Verification items for this drawing (mm, ordinates from the low corner). Coordinates: 2 decimals unless noted, no trailing zeros. Write each loop counter-clockwise with the first axis right and the second up, starting at its lowest first coordinate (ties: lowest second). Pieces come first, ordered by that corner, then holes. Notation, with made-up numbers: (58.5, -21) -> (89.5, -21) arc R26 ccw to (89.5, 7) -> close; hole circle Ø6 at (-15.5, 39). An arc over 180 degrees is marked (long way). Put each result on its own line as item: value. Start each with the question number.
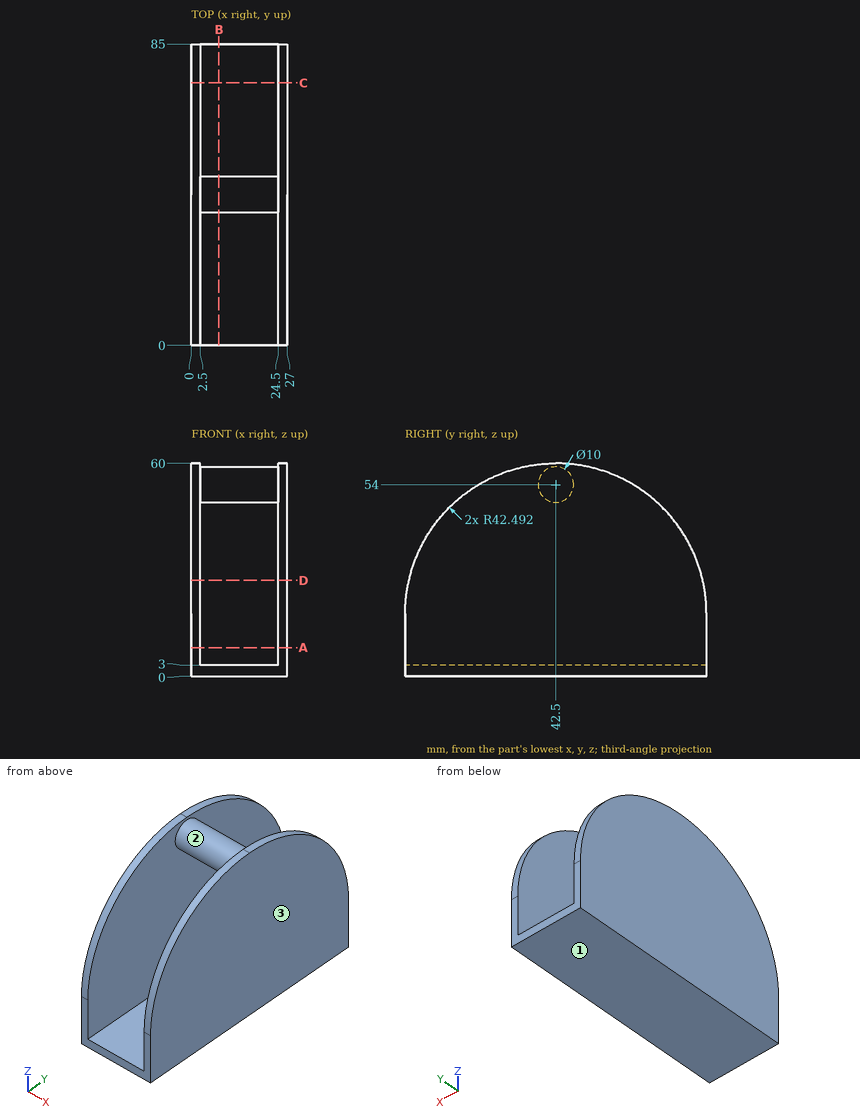
Item 1: Mould release check, pull along Z, two halves, no side actions. Record for the marked faces 1, 2 and 3: released by +Z, released by -Z, zero draft, split by the parting line, or undercut.
Item 2: Scan lines: line 1 along X through (y, z) = (31.5, 54.5); line 2 along Z through (x, y) = (19, 14.5); line 3 along Z through (x, y) = (6.75, 44). Record each from-to range of solid material in increasing order. Write a range as [from, to].
Item 3: Section check D-D, the plane z = 27. Enter the section's corners in (x, y).
Item 4: Section check A-A, the plane z = 8. Enter the section's corners in (x, y), and give its area (3 significant figures).
Item 5: Section check C-C, the plane y = 74. Enter the section's corners in (x, z) (1 decimal), and give its area (3 significant figures).
Item 6: Section check B-B, the plane x = 7.75. Enter the section's corners in (y, z).
Item 7: Go/stop test with flat-tipped pins: P1, Ø1.5, axis at x = 9, z = 53.5, coming from the +Y side; P2, Ø8, axis at y = 24, z = 15, coming from the -X side; P3, Ø12, axis at x = 5.5, y = 13.5, coming from the +Z side; P4, Ø11, axis at x = 16.5, y = 38.5, coming from the +Z side. Record where each tip stops, or that it passes through.
From the geometry:
1. face 1: released by -Z
1. face 2: undercut
1. face 3: zero draft
2. line 1: [0, 2.5], [24.5, 27]
2. line 2: [0, 3]
2. line 3: [0, 3], [49.23, 58.77]
3. outline: (0, 1.07) -> (2.5, 1.07) -> (2.5, 83.93) -> (0, 83.93) -> close; (24.5, 1.07) -> (27, 1.07) -> (27, 83.93) -> (24.5, 83.93) -> close
4. outline: (0, 0) -> (2.5, 0) -> (2.5, 85) -> (0, 85) -> close; (24.5, 0) -> (27, 0) -> (27, 85) -> (24.5, 85) -> close
4. area: 425 mm²
5. outline: (0, 0) -> (27, 0) -> (27, 46) -> (24.5, 46) -> (24.5, 3) -> (2.5, 3) -> (2.5, 46) -> (0, 46) -> close
5. area: 296 mm²
6. outline: (0, 0) -> (85, 0) -> (85, 3) -> (0, 3) -> close; circle Ø10 at (42.5, 54)
7. P1: y = 47.5
7. P2: x = 0
7. P3: z = 52.71
7. P4: z = 59
